Design review of the part built by this model. Coordinates are the model's own, in mm. A direction names the side the tool comes from. Give positions to 0.01 mm unless a question says otherwise; leave off trailing zeros. Write each loop counter-clockwise with the first axis right and the second up, starting at its lowest first coordinate (ties: lowest second). Pieces come first, ordered by that corner, then holes. Notation, with made-up numbers: (40, 17.25) - (90, 17.25) arc R5 cw to (90, 25.25) - close; hole circle Ø8 at (-16.5, -21). An arc over 180 degrees is marked (long way). Use a Markdown table: item, result. Add a question column.
```python
from build123d import *

# Parameters (mm, degrees)
EXTRUDE_1_DEPTH     = 10
SKETCH_2_W          = 4
SKETCH_2_H          = 30
EXTRUDE_3_DEPTH     = 40
CUT_EXTRUDE_1_DEPTH = 123.474487139


with BuildPart() as part:
    # 草图1 → 凸台-拉伸1 (new body)
    with BuildSketch(Plane(origin=(0, 0, 0), x_dir=(0, 0, -1), z_dir=(1, 0, 0))):
        with BuildLine():
            Line((-50, 30), (-46, 30))
            Line((-46, 30), (-46, 19.595917942))
            ThreePointArc((-46, 19.595917942), (0, 50), (46, 19.595917942))
            Line((46, 19.595917942), (46, 30))
            Line((46, 30), (50, 30))
            Line((50, 30), (50, -30))
            Line((50, -30), (46, -30))
            Line((46, -30), (46, 0))
            ThreePointArc((46, 0), (0, 46), (-46, 0))
            Line((-46, 0), (-46, -30))
            Line((-46, -30), (-50, -30))
            Line((-50, -30), (-50, 30))
        make_face()
    extrude(amount=EXTRUDE_1_DEPTH)

    # 草图2 → 凸台-拉伸3 (add)
    with BuildSketch(Plane(origin=(10, 0, 0), x_dir=(0, 0, -1), z_dir=(1, 0, 0))):
        with Locations((-48, -15)):
            Rectangle(SKETCH_2_W, SKETCH_2_H)
        with Locations((48, -15)):
            Rectangle(SKETCH_2_W, SKETCH_2_H)
    extrude(amount=EXTRUDE_3_DEPTH)

    # 草图3 → 切除-拉伸1 (cut, through all)
    with BuildSketch(Plane(origin=(0, 0, -50), x_dir=(-1, 0, 0), z_dir=(0, 0, -1))):
        with BuildLine():
            Line((-42, -15), (-42, -32.28163942))
            Line((-42, -32.28163942), (-57, -32.28163942))
            Line((-57, -32.28163942), (-57, -30))
            ThreePointArc((-57, -30), (-67.606601718, -4.393398282), (-42, -15))
        make_face()
    extrude(amount=-CUT_EXTRUDE_1_DEPTH, mode=Mode.SUBTRACT)


solid = part.part
```
(1) Add section B-B (y = 3). State the section outline as (x, z) points.
(2) Add section A-A (x = 16.5). State the section outline as (y, z) points, and give its area (3 significant figures).
(3) Tool access review of faces 4 (the face through (25, -15, 46)), 5 (the face through (30, 0, -48)), 6 (the face through (42, -22, -48)), 7 (the face through (5, 30, -48)): name each direction out of +Z, -Z, +X, -X, +Y, -Y from which nothing blocks a thin tool from reaching the whole face with its end or side.
(4) Mouldability with a two-part tool opening along Z and no side actions: class faces 1 (the face through (19, -6, -50)), 2 (the face through (5, 25, 46)), 3 (the face through (21, -30, 48)) as +Z half, -Z half, draft (parallel to the pull), parting line (faces both ways), or undercut.
(5) For line 1 along Z through (x, y) = (19, -11); line 2 along Y through (x, z) = (4, -28); line 3 along Y through (x, z) = (6.5, -11) (3 decimals), list the stretches that pass through material, from the lowest coordinate up.
(6) Insertion check: pin 1 (2 mm diameter, centred on x = 5.5, z = -35, fed in from +Y); pin 2 (3 mm diameter, centred on x = 35.5, z = -47.5, fed in from +Y); pin 3 (4.5 mm diameter, centred on y = -22, z = -48.5, fed in from +X). Each pin has a flat end and moves straight along its axis. Give the tip position at first contact, or say it passes through.
(7) Add section D-D (z = -37). State the section outline as (x, y) points.
(8) Add section C-C (z = 0). State the section outline as (x, y) points.
Answers follow:
| question | item | result |
|---|---|---|
| 1 | outline | (0, -50) - (10, -50) - (10, -45.9) - (0, -45.9) - close; (0, 45.9) - (10, 45.9) - (10, 50) - (0, 50) - close |
| 2 | outline | (-30, -50) - (0, -50) - (0, -46) - (-30, -46) - close; (-30, 46) - (0, 46) - (0, 50) - (-30, 50) - close |
| 2 | area | 240 mm^2 |
| 3 | face 4 | +X, -X, -Y |
| 3 | face 5 | +Z, -Z, +X, +Y |
| 3 | face 6 | +Z, -Z, +X, -Y |
| 3 | face 7 | -Z, +X, -X, +Y |
| 4 | face 1 | -Z half |
| 4 | face 2 | undercut |
| 4 | face 3 | draft |
| 5 | line 1 | -50 to -46, 46 to 50 |
| 5 | line 2 | 36.5 to 41.42 |
| 5 | line 3 | 44.665 to 48.775 |
| 6 | pin 1 | y = 36.66 |
| 6 | pin 2 | y = 0 |
| 6 | pin 3 | x = 42 |
| 7 | outline | (0, 27.33) - (10, 27.33) - (10, 33.63) - (0, 33.63) - close |
| 8 | outline | (0, 46) - (10, 46) - (10, 50) - (0, 50) - close |
